Read the model definition and answer for the solid it produces. Units are mm, in the model's axes. A direction names the side the tool comes from. Give positions to 0.01 mm unless a question says otherwise; leave off trailing zeros. Order: outer loops, then holes, each group sorted by start corner. A loop starts at its lowest first (then second) coordinate and runs counter-clockwise, first axis right, second up.
Item 1: The mould has two halves that part along Z. Classify faces 1 (the face through (337.421, -189.482, -2486.183)), 2 (the face through (416.534, -155.183, -2193.119)), 3 (the face through (330, -41.582, -2493)): +Z half, -Z half, draft (parallel to the pull), parting line (faces both ways), or undercut.
Item 2: Find the intervals of material crossed by line 1 along X through (y, z) = (-191, -2458); line 2 along X through (y, z) = (-242.5, -2641), in increasing order.
Item 3: Which of the six approach directions +Z, -Z, +X, -X, +Y, -Y give full straight-line access (tool end or side, diameter ignored) to faces 4 (the face through (246, -154.082, -2785)), 5 (the face through (246, -229.082, -2785)), 6 (the face through (416.58, -230.28, -2192.96))?
Item 4: Given pin 1 Ø10.5 at (x, z) = (244.5, -2784.5) entering from -Y; pin 2 Ø1 at (y, z) = (-269, -2499) entering from +X; pin 3 Ø1 at (y, z) = (-284, -2726.5) entering from +X, each flat-ended and moving along its own axis, determine where each tip first touches the part or whether it passes through.
Item 5: A cutting plane is placed at B-B (z = -2268.5). Write down the section's boundary in (x, y), plus the area to 3 significant figures.
Item 6: A cutting plane is placed at A-A (y = -263.5). Write down the section's boundary in (x, z).
from build123d import *

# Parameters (mm, degrees)
BOSS_EXTRUDE1_DEPTH = 10.16


with BuildPart() as part:
    # Sketch1 → Boss-Extrude1 (new body)
    with BuildSketch(Plane(origin=(972.287594707, 0, -279.761907089), x_dir=(-0.27651668570360943, 0, -0.9610091167764702), z_dir=(0.9610091167764702, 0, -0.27651668570360943))):
        Polygon((2602.330216376, -41.581628832), (1998.345068474, -41.581628832), (1998.345068474, -156.254177234), (1986.345068474, -154.081628832), (1986.345068474, -229.081628832), (1998.345068474, -231.512401326), (1998.345068474, -341.581628832), (2602.330216376, -341.581628832), (2602.330216376, -229.081628832), (2614.330216376, -229.081628832), (2614.330216376, -154.081628832), (2602.330216376, -154.081628832), align=None)
    extrude(amount=-BOSS_EXTRUDE1_DEPTH)


solid = part.part
Response values:
1. face 1: -Z half
1. face 2: undercut
1. face 3: draft
2. line 1: x = 334.96 to 345.53
2. line 2: x = 282.3 to 292.87
3. face 4: -Z, -X, +Y
3. face 5: -Z, -X, -Y
3. face 6: +Z, +X, -Y
4. pin 1: stops at y = -229.08
4. pin 2: stops at x = 333.88
4. pin 3: stops at x = 268.42
5. outline: (389.48, -341.58) - (400.06, -341.58) - (400.06, -41.58) - (389.48, -41.58) - close
5. area: 3,170 mm2
6. outline: (242.94, -2777.82) - (252.7, -2780.62) - (419.71, -2200.19) - (409.95, -2197.38) - close
